Model file for the job. Use its own axes, mm. Face numbers are marked on the shaded views. A direction names the side the tool comes from. Coordinates: 2 decimals unless noted, no trailing zeros. Loops run counter-clockwise (first coordinate to the right, second up) from the corner with the lowest first, then second, coordinate; pieces in that order, holes last. Notation, with made-up numbers: (20.25, 85.5) - (40.25, 85.5) arc R21 ccw to (40.25, 111.5) - close; hole circle Ø11 at (-35, 77). An arc over 180 degrees is marked (long way). Write each question's results on one line, items separated by ' | '. Start each with the question number.
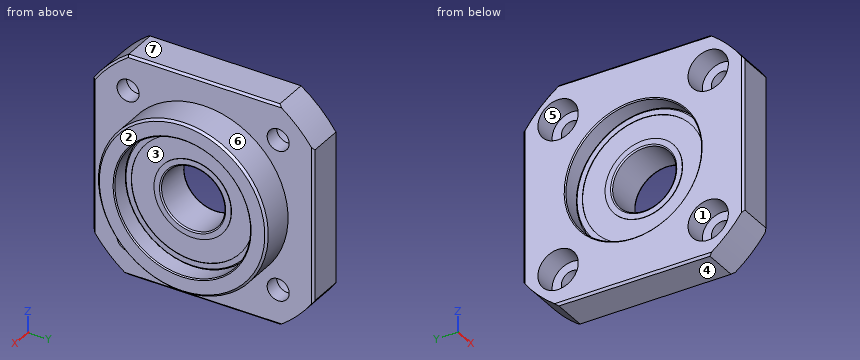
```python
from build123d import *

# Parameters (mm, degrees)
SKIZZE1_W                       = 52
SKIZZE1_H                       = 52
AUFSATZ_LINEAR_AUSTRAGEN1_DEPTH = 17
SKIZZE2_R                       = 63
SKIZZE2_R_2                     = 31.5
SCHNITT_LINEAR_AUSTRAGEN1_DEPTH = 17
SKIZZE3_R                       = 63
SKIZZE3_R_2                     = 20
SCHNITT_LINEAR_AUSTRAGEN2_DEPTH = 8
SKIZZE4_R                       = 16
SCHNITT_LINEAR_AUSTRAGEN3_DEPTH = 17
SKIZZE5_R                       = 2.6
SCHNITT_LINEAR_AUSTRAGEN4_DEPTH = 9
LINEARES_MUSTER1_COUNT          = 2
LINEARES_MUSTER1_PITCH          = 35.355339059
LINEARES_MUSTER1_COUNT_DIR2     = 2
LINEARES_MUSTER1_PITCH_DIR2     = 35.355339059
SKIZZE7_R                       = 4.75
SCHNITT_LINEAR_AUSTRAGEN5_DEPTH = 5.4
LINEARES_MUSTER2_COUNT          = 2
LINEARES_MUSTER2_PITCH          = 35.355339059
LINEARES_MUSTER2_COUNT_DIR2     = 2
LINEARES_MUSTER2_PITCH_DIR2     = 35.355339059
FASE1_SIZE                      = 0.5
FASE2_SIZE                      = 0.5
FASE3_SIZE                      = 0.25


with BuildPart() as part:
    # Skizze1 → Aufsatz-Linear austragen1 (new body)
    with BuildSketch(Plane(origin=(0, 0, 0), x_dir=(0, 0, -1), z_dir=(1, 0, 0))):
        Rectangle(SKIZZE1_W, SKIZZE1_H)
    extrude(amount=AUFSATZ_LINEAR_AUSTRAGEN1_DEPTH)

    # Skizze2 → Schnitt-Linear austragen1 (cut)
    with BuildSketch(Plane(origin=(0, 0, 0), x_dir=(0, 0, -1), z_dir=(1, 0, 0))):
        Circle(SKIZZE2_R)
        Circle(SKIZZE2_R_2, mode=Mode.SUBTRACT)
    extrude(amount=SCHNITT_LINEAR_AUSTRAGEN1_DEPTH, mode=Mode.SUBTRACT)

    # Skizze3 → Schnitt-Linear austragen2 (cut)
    with BuildSketch(Plane(origin=(9, 0, 0), x_dir=(0, 0, -1), z_dir=(1, 0, 0))):
        Circle(SKIZZE3_R)
        Circle(SKIZZE3_R_2, mode=Mode.SUBTRACT)
    extrude(amount=SCHNITT_LINEAR_AUSTRAGEN2_DEPTH, mode=Mode.SUBTRACT)

    # Skizze4 → Schnitt-Linear austragen3 (cut)
    with BuildSketch(Plane(origin=(0, 0, 0), x_dir=(0, 0, -1), z_dir=(1, 0, 0))):
        Circle(SKIZZE4_R)
    extrude(amount=SCHNITT_LINEAR_AUSTRAGEN3_DEPTH, mode=Mode.SUBTRACT)

    # Skizze5 → Schnitt-Linear austragen4 (cut)
    with BuildSketch(Plane(origin=(0, 0, 0), x_dir=(0, 0, -1), z_dir=(1, 0, 0))):
        with Locations((-17.67766953, 17.67766953)):
            Circle(SKIZZE5_R)
    schnitt_linear_austragen4 = extrude(amount=SCHNITT_LINEAR_AUSTRAGEN4_DEPTH, mode=Mode.SUBTRACT)

    # Lineares Muster1: Schnitt-Linear austragen4 2 × 2
    with Locations(*[(0, -j * LINEARES_MUSTER1_PITCH_DIR2, -i * LINEARES_MUSTER1_PITCH) for i in range(LINEARES_MUSTER1_COUNT) for j in range(LINEARES_MUSTER1_COUNT_DIR2) if (i, j) != (0, 0)]):
        add(schnitt_linear_austragen4, mode=Mode.SUBTRACT)

    # Skizze7 → Schnitt-Linear austragen5 (cut)
    with BuildSketch(Plane(origin=(0, 0, 0), x_dir=(0, 0, -1), z_dir=(1, 0, 0))):
        with Locations((-17.67766953, 17.67766953)):
            Circle(SKIZZE7_R)
    schnitt_linear_austragen5 = extrude(amount=SCHNITT_LINEAR_AUSTRAGEN5_DEPTH, mode=Mode.SUBTRACT)

    # Lineares Muster2: Schnitt-Linear austragen5 2 × 2
    with Locations(*[(0, -j * LINEARES_MUSTER2_PITCH_DIR2, -i * LINEARES_MUSTER2_PITCH) for i in range(LINEARES_MUSTER2_COUNT) for j in range(LINEARES_MUSTER2_COUNT_DIR2) if (i, j) != (0, 0)]):
        add(schnitt_linear_austragen5, mode=Mode.SUBTRACT)

    # Skizze9 → Rotation1 (revolve)
    with BuildSketch(Plane(origin=(0, 0, 0), x_dir=(-1, 0, 0), z_dir=(0, 0, -1)), mode=Mode.PRIVATE) as rotation1_sk:
        with BuildLine():
            Line((-13, 15.7), (-13, 14.45))
            Line((-13, 14.45), (-12.9, 14.45))
            Line((-12.9, 14.45), (-12.9, 9.1))
            Line((-12.9, 9.1), (-13, 9.1))
            Line((-13, 9.1), (-13, 7.8))
            ThreePointArc((-13, 7.8), (-12.912132034, 7.587867966), (-12.7, 7.5))
            Line((-12.7, 7.5), (-4.3, 7.5))
            ThreePointArc((-4.3, 7.5), (-4.087867966, 7.587867966), (-4, 7.8))
            Line((-4, 7.8), (-4, 9.1))
            Line((-4, 9.1), (-4.1, 9.1))
            Line((-4.1, 9.1), (-4.1, 14.45))
            Line((-4.1, 14.45), (-4, 14.45))
            Line((-4, 14.45), (-4, 15.7))
            ThreePointArc((-4, 15.7), (-4.087867966, 15.912132034), (-4.3, 16))
            Line((-4.3, 16), (-12.7, 16))
            ThreePointArc((-12.7, 16), (-12.912132034, 15.912132034), (-13, 15.7))
        make_face()
    revolve(rotation1_sk.sketch.rotate(Axis((-500, 0, 0), (1, 0, 0)), 270), axis=Axis((-500, 0, 0), (1, 0, 0)))  # turned: the seam where the file's is

    # Fase1
    fase1_edges = [part.edges().sort_by_distance(p)[0] for p in [
        (17, 0, 20),
    ]]
    chamfer(fase1_edges, length=FASE1_SIZE)

    # Fase2
    fase2_edges = [part.edges().sort_by_distance(p)[0] for p in [
        (0, -26, 0),
        (0, 0, -26),
        (9, 0, 26),
        (9, -22.273863607, 22.273863607),
        (9, -26, 0),
        (9, 0, -26),
        (9, 26, 0),
        (0, 0, 26),
        (0, 26, 0),
        (0, 22.273863607, 22.273863607),
    ]]
    chamfer(fase2_edges, length=FASE2_SIZE)

    # Fase3
    fase3_edges = [part.edges().sort_by_distance(p)[0] for p in [
        (0, 0, 16),
        (17, 0, 16),
    ]]
    chamfer(fase3_edges, length=FASE3_SIZE)


solid = part.part
```
Q1. Which spindle directions (+Z, -Z, +X, -X, +Y, -Y) get a long thin tool onto all of the face, cutting with end or side? Do the marked faces 1, 2 and 3. Say none if no direction does.
Q2. Drill centre lines: L1, parallel to Z at x = 7.75, y = -18.5; L2, parallel to X at y = -11, z = -9; L3, parallel to Y at x = 15.85, z = 0. Where is each one in solid material? Low to high. Write a range as from..to.
Q3. Mould opens along Z. For the marked faces 4, 5, 6 and 7 say: +Z half, -Z half, draft (parallel to the pull), parting line (faces both ways), or undercut.
Q4. Cut at A-A (x = 14.75). List the corners of the cut face in (y, z), and give its area (3 significant figures).
Q5. Pin check, flat tips, straight feed: pin 1 (8.5 mm diameter, centred on y = 17.68, z = 17.68, fed in from +X); pin 2 (20 mm diameter, centred on y = -1, z = -1.5, fed in from -X); pin 3 (5 mm diameter, centred on y = -19.5, z = 18.5, fed in from -X). Stop position of each tip, or through.
Check result:
1) face 1: -X | face 2: +Z, -Z, +X, +Y, -Y | face 3: +X
2) L1: -25.5..-20.14, -15.21..15.21, 20.14..25.5 | L2: 4.1..12.9 | L3: -20..-16, 16..20
3) face 4: -Z half | face 5: undercut | face 6: parting line | face 7: +Z half
4) outline: circle Ø40 at (0, 0); hole circle Ø32 at (0, 0) | area: 452 mm²
5) pin 1: x = 9 | pin 2: x = 4 | pin 3: x = 5.4
